Part model, mm, in its own coordinate system. A direction names the side the tool comes from. Round coordinates to 2 decimals unless told otherwise and drop trailing zeros. Write each loop counter-clockwise with the first axis right and the second up, starting at its lowest first coordinate (ties: lowest second). Pieces come first, ordered by that corner, then holes.
Autodesk Inventor part; units mm, degrees
ref_plane "YZ Plane" through (0, 0, 0) normal (1, 0, 0) x (0, 1, 0)
ref_plane "XZ Plane" through (0, 0, 0) normal (0, 1, 0) x (-1, 0, 0)
ref_plane "XY Plane" through (0, 0, 0) normal (0, 0, 1) x (1, 0, 0)
sketch "Sketch1" plane through (0, 0, 0) normal (0, 1, 0) x (-1, 0, 0)
  line L0 (0, 3.1877) -> (3.1877, 3.1877)
  line L1 (3.1877, 3.1877) -> (3.1877, -3.175)
  line L2 (3.1877, -3.175) -> (0, -3.175)
  line L3 (0, 5.08) -> (5.08, 5.08)
  line L4 (5.08, 5.08) -> (5.08, -5.08)
  line L5 (5.08, -5.08) -> (0, -5.08)
  line L6 (0, -5.08) -> (0, -3.175)
  line L7 (0, 3.1877) -> (0, 5.08)
  point P0 (0, 0)
  dimension "d0" = 3.1877
  dimension "d1" = 5.08
  dimension "d2" = 10.16
extrude "Extrusion1" add sketch "Sketch1" along normal blind 85.4964
sketch "Sketch2" plane through (0, 85.4964, 0) normal (0, 1, 0) x (1, 0, 0)
  line L0 (0, -5.08) -> (0, -3.1877)
  line L1 (0, 5.08) -> (-5.08, 5.08)
  line L2 (0, -5.08) -> (-5.08, -5.08)
  line L3 (-5.08, -5.08) -> (-5.08, 5.08)
  line L4 (-5.08, 5.08) -> (0, 5.08)
  line L5 (0, 5.08) -> (0, -5.08)
  point P0 (0, 0)
extrude "Extrusion2" add sketch "Sketch2" along normal blind 1.8923
sketch "Sketch3" plane through (-5.08, 0, -5.08) normal (-1, 0, 0) x (0, 0, 1)
  circle A0 centre (5.08, 5.4991) radius 1.9844
  circle A1 centre (5.08, 79.9973) radius 1.9844
  point P0 (5.08, 0)
  dimension "d7" = 3.9688
  dimension "d8" = 3.9688
extrude "Extrusion3" cut sketch "Sketch3" against normal blind 1.8923
sketch "Sketch4" plane through (-5.08, 5.4991, 0) normal (-1, 0, 0) x (0, 0, 1)
  circle A0 centre (0, 0) radius 1.9844
  circle A1 centre (0, 0) radius 1.9844
  circle A2 centre (0, 0) radius 5.08
  line L0 (5.08, -5.4991) -> (5.08, 81.8896)
  circle A3 centre (0, 74.4982) radius 1.9844
  circle A4 centre (0, 74.4982) radius 1.9844
  circle A5 centre (0, 74.4982) radius 5.08
  point P0 (0, -5.4991)
extrude "Extrusion4" add sketch "Sketch4" along normal blind 9.525
properties part number "hs_intake_joint"
Q1. Cut at A-A on z = 0. Write the cut outline in (x, y) (1 decimal).
Values follow:
outline: (-14.6, 0.4) - (-5.1, 0.4) - (-5.1, 0) - (-3.2, 0) - (-3.2, 3.5) - (-14.6, 3.5) - close; (-14.6, 7.5) - (-3.2, 7.5) - (-3.2, 78) - (-14.6, 78) - (-14.6, 74.9) - (-5.1, 74.9) - (-5.1, 10.6) - (-14.6, 10.6) - close; (-14.6, 82) - (-3.2, 82) - (-3.2, 85.5) - (0, 85.5) - (0, 87.4) - (-5.1, 87.4) - (-5.1, 85.1) - (-14.6, 85.1) - close
Q2. Wall check: L1, parallel to Y at x = -9, z = 0; L2, parallel to Y at x = -3.5, z = 1; L3, parallel to Y at x = -6.5, z = -1.75. Give the ranges that are in metal, low to high.
Values follow:
L1: y = 0.42 to 3.51, 7.48 to 10.58, 74.92 to 78.01, 81.98 to 85.08
L2: y = 0 to 3.79, 7.21 to 78.28, 81.71 to 87.39
L3: y = 0.73 to 4.56, 6.43 to 10.27, 75.23 to 79.06, 80.93 to 84.77
Q3. Drop flat-ended pins along their axis: pin 1 (2.5 mm diameter, centred on x = -2, z = -1, fed in from -Y); pin 2 (1.5 mm diameter, centred on x = -10, z = -2, fed in from -Y); pin 3 (1.5 mm diameter, centred on y = 36, z = -1, fed in from +X); pin 4 (8 mm diameter, centred on x = -12, y = 24.5, fed in from +Z). Give the stop position or say it passes through.
Values follow:
pin 1: stops at y = 0
pin 2: stops at y = 0.58
pin 3: stops at x = -3.19
pin 4: passes through
Q4. Mould opens along Z. For faces 1 (the flat face through (-3, 43, -5.08)), 2 (the flat face through (-5.08, 0.3, -0.7)), 3 (the flat face through (-2, 42, -3.175)) say: +Z half, -Z half, draft (parallel to the pull), parting line (faces both ways), or undercut.
Values follow:
face 1: -Z half
face 2: draft
face 3: undercut
Q5. Cut at C-C on y = 39. Write the cut outline in (x, z) (3 decimals), plus the area to 3 significant figures.
Values follow:
outline: (-5.08, -5.08) - (0, -5.08) - (0, -3.175) - (-3.188, -3.175) - (-3.188, 3.188) - (0, 3.188) - (0, 5.08) - (-5.08, 5.08) - close
area: 31.3 mm2
Q6. Which spindle directions (+Z, -Z, +X, -X, +Y, -Y) get a long thin tool onto all of the face, cutting with end or side? Do faces 4 (the cylindrical face through (-9.776, 0.462, -0.661)), 5 (the flat face through (-2, 85.496, 0)), 6 (the flat face through (-14.605, 80.1, 2.2)). Say none if no direction does.
Values follow:
face 4: -X
face 5: +X, -Y
face 6: +Z, -Z, -X, +Y, -Y
Q7. Cut at B-B on x = -8.5. Write the cut outline in (y, z), plus the area to 3 significant figures.
Values follow:
outline: circle Ø10.16 at (5.5, 0); circle Ø10.16 at (80, 0); hole circle Ø3.97 at (5.5, 0); hole circle Ø3.97 at (80, 0)
area: 137 mm2
